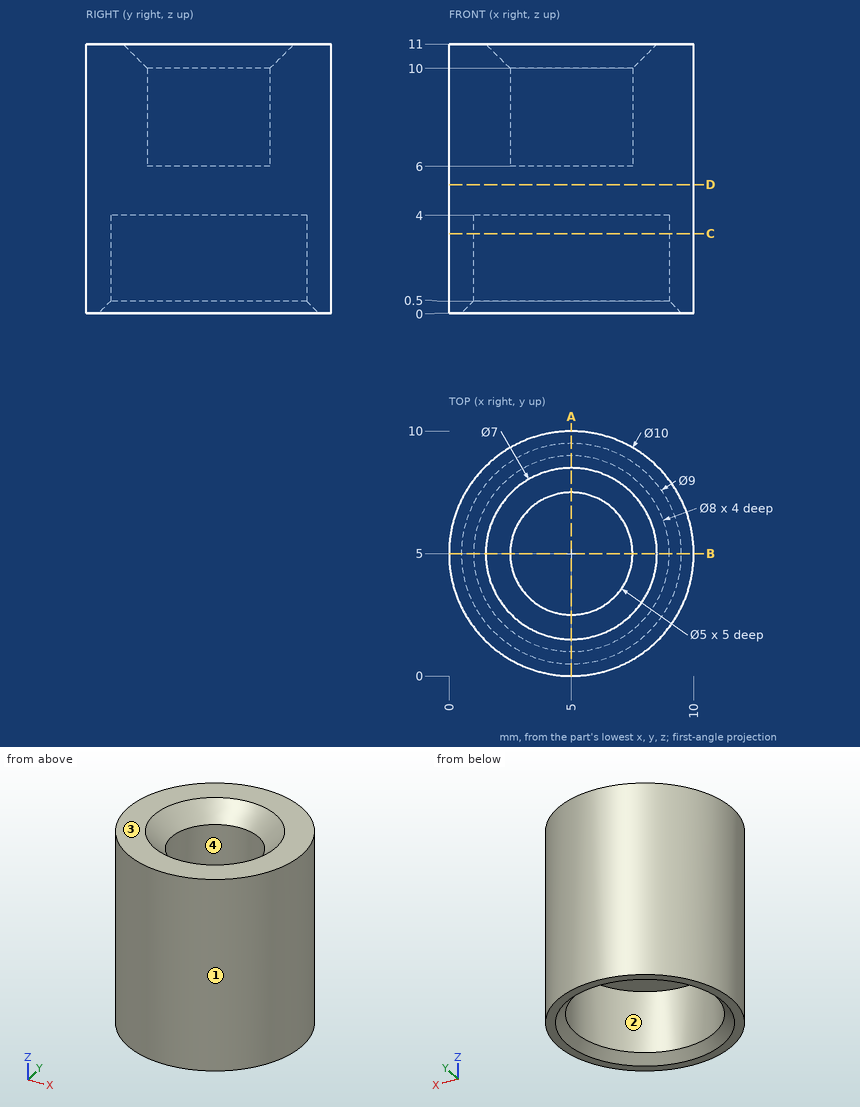
Could you check a few things on this drawing? It's one solid part, dimensions in mm from its lowest x, y, z. Coordinates: 2 decimals unless noted, no trailing zeros. Order: outer loops, then holes, each group sorted by start corner. A loop starts at its lowest first (then second) coordinate and runs counter-clockwise, first axis right, second up. Notation, with made-up numbers: (71.25, 45) - (84.25, 45) arc R17 ccw to (84.25, 58) - close; hole circle Ø7 at (83, 67). An arc over 180 degrees is marked (long way). One line per question, with ' | ' between items. Start each with the question number.
1. If we section it at A-A (x = 5): Write out the boundary of the cut face in (y, z), and give its area (4 significant figures).
2. Please list where these lines run through material, in increasing order: line 1 along Y through (x, z) = (5, 8.9); line 2 along Y through (x, z) = (5, 2.5); line 3 along Z through (x, y) = (5.5, 5.75). Write a range as [from, to].
3. If we section it at D-D (z = 5.25): Write out the boundary of the cut face in (x, y), and give its area (3 significant figures).
4. If we section it at C-C (z = 3.25): Write out the boundary of the cut face in (x, y).
5. If we mould it in two halves opening along Y, with no side actions, what happens to the marked faces 1, 2, 3 and 4? For each: released by +Y, released by -Y, zero draft, split by the parting line, or undercut.
6. I'm going to push flat-ended pins straight in: pin 1 Ø3 at (y, z) = (1.5, 1) entering from +X; pin 2 Ø3 at (x, y) = (5, 5) entering from +Z; pin 3 Ø5 at (x, z) = (8, 7) entering from +Y. Where does each tip first touch, or does it pass through?
Model answer:
1) outline: (0, 0) - (0.5, 0) - (1, 0.5) - (1, 4) - (9, 4) - (9, 0.5) - (9.5, 0) - (10, 0) - (10, 11) - (8.5, 11) - (7.5, 10) - (7.5, 6) - (2.5, 6) - (2.5, 10) - (1.5, 11) - (0, 11) - close | area: 51.75 mm²
2) line 1: y = [0, 2.5], [7.5, 10] | line 2: y = [0, 1], [9, 10] | line 3: z = [4, 6]
3) outline: circle Ø10 at (5, 5) | area: 78.5 mm²
4) outline: circle Ø10 at (5, 5); hole circle Ø8 at (5, 5)
5) face 1: split by the parting line | face 2: undercut | face 3: zero draft | face 4: undercut
6) pin 1: stops at x = 9.58 | pin 2: stops at z = 6 | pin 3: stops at y = 9.97
